Input: dimensioned drawing with shaded views. Units: mm. Origin: part minimum x, y, z. Give positions to 0.01 mm unless a question says otherwise; leave off trailing zeros. Order: outer loops, then holes, each group sorted by start corner. A loop starts at its lowest first (then second) coordinate and runs counter-clockwise, first axis right, second up. Notation, with made-up numbers: (38, -6) -> (56, -6) arc R20 cw to (56, 26) -> close; hole circle Ø3 at (-27, 3). An arc over 180 degrees is marked (long way). One line per question, with ' | ' between items. Start each with the question number.
(1) Ray query, L1, parallel to X at y = 462.5, z = 149; L2, parallel to Z at x = 121.5, y = 532; L3, parallel to Z at x = 639.5, y = 306.5. Return the intervals inside material, ascending.
(2) First-contact query: pin 1 Ø12 at (x, y) = (452.5, 82) entering from +Z; pin 2 Ø10 at (x, y) = (236, 546) entering from -Z; pin 3 Ø3 at (x, z) = (821.5, 559.5) entering from +Y. Flat tips, straight axial feed; report the tip coordinate or a pass-through.
(3) Section C-C (x = 527). Return loops of the section in (y, z).
(4) Section B-B (y = 299.5). Return loops of the section in (x, z), then the cut area to 3 significant figures.
(5) Section A-A (z = 344). Return loops of the section in (x, y).
(6) Section D-D (z = 765). Return loops of the section in (x, y).
(7) Mould query, pull axis X, two halves, no side actions, for the marked faces 1, 2 and 3. Classes: +X half, -X half, draft (parallel to the pull), parting line (faces both ways), or undercut.
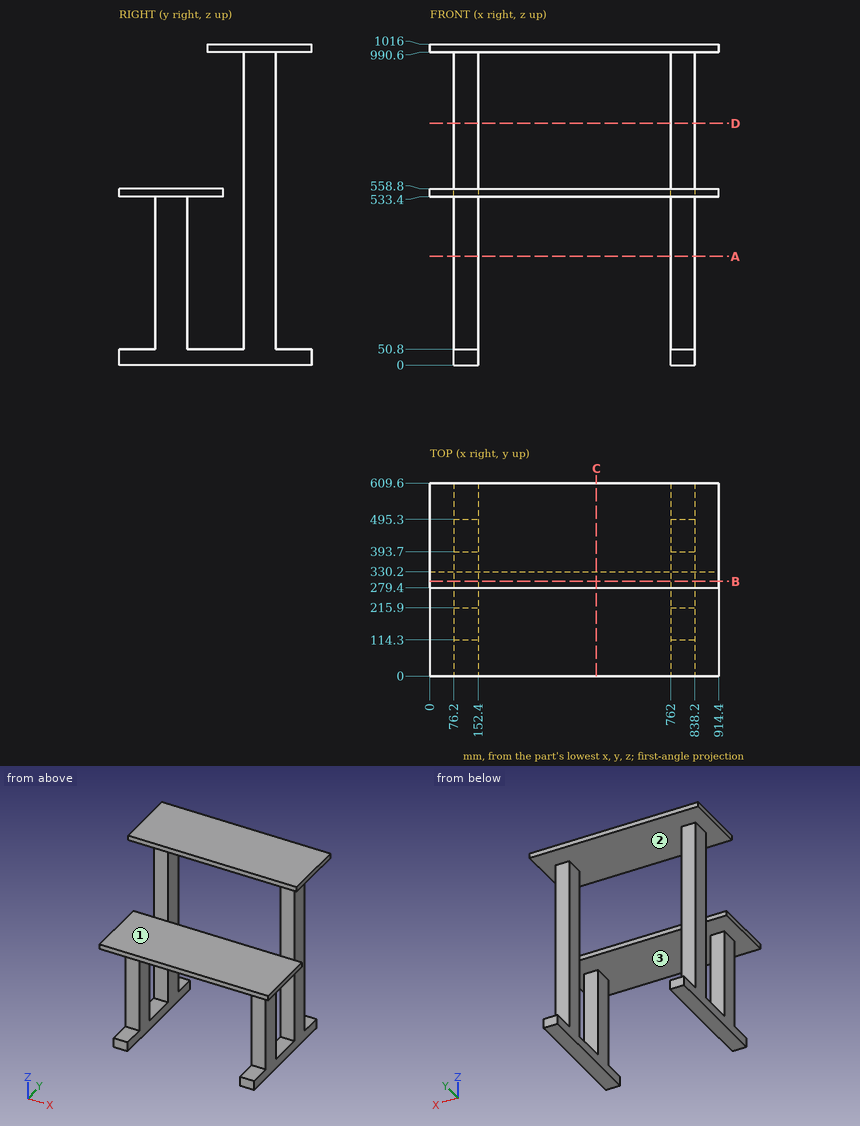
Response:
1) L1: x = 76.2 to 152.4, 762 to 838.2 | L2: z = 0 to 50.8, 990.6 to 1016 | L3: z = 533.4 to 558.8, 990.6 to 1016
2) pin 1: stops at z = 558.8 | pin 2: stops at z = 990.6 | pin 3: stops at y = 495.3
3) outline: (0, 533.4) -> (330.2, 533.4) -> (330.2, 558.8) -> (0, 558.8) -> close; (279.4, 990.6) -> (609.6, 990.6) -> (609.6, 1016) -> (279.4, 1016) -> close
4) outline: (0, 533.4) -> (914.4, 533.4) -> (914.4, 558.8) -> (0, 558.8) -> close; (0, 990.6) -> (914.4, 990.6) -> (914.4, 1016) -> (0, 1016) -> close; (76.2, 0) -> (152.4, 0) -> (152.4, 50.8) -> (76.2, 50.8) -> close; (762, 0) -> (838.2, 0) -> (838.2, 50.8) -> (762, 50.8) -> close | area: 54,200 mm^2
5) outline: (76.2, 114.3) -> (152.4, 114.3) -> (152.4, 215.9) -> (76.2, 215.9) -> close; (76.2, 393.7) -> (152.4, 393.7) -> (152.4, 495.3) -> (76.2, 495.3) -> close; (762, 114.3) -> (838.2, 114.3) -> (838.2, 215.9) -> (762, 215.9) -> close; (762, 393.7) -> (838.2, 393.7) -> (838.2, 495.3) -> (762, 495.3) -> close
6) outline: (76.2, 393.7) -> (152.4, 393.7) -> (152.4, 495.3) -> (76.2, 495.3) -> close; (762, 393.7) -> (838.2, 393.7) -> (838.2, 495.3) -> (762, 495.3) -> close
7) face 1: draft | face 2: undercut | face 3: undercut
